Can you work these out from the model? Positions are in its coordinate system, mm. A direction names the side the tool comes from. Coordinates: 2 decimals unless noted, no trailing zeros. Order: outer loops, then holes, each group sorted by start corner. A loop starts at its lowest first (then second) coordinate and runs counter-clockwise, first axis right, second up. Notation, with made-up numbers: (65, 34.25) - (107, 34.25) arc R35 cw to (107, 73.25) - close; hole circle Ø5 at (38.25, 6.25). An arc over 180 degrees is marked (long way). Use a Markdown table: item, result. Add a question column.
(1) We'd pull the mould along X, two halves only. Please class faces 5 (the flat face through (0, -6, 16.51)), 6 (the flat face through (0, 0, 13.97)), 7 (the cylindrical face through (6.49, -10.17, 6.89)), 8 (the cylindrical face through (-1.86, -14.166, 8.139)): pulls with the +X half, pulls with the -X half, needs draft (parallel to the pull), parting line crosses it, or undercut.
(2) I want a section at A-A (x = 0). State how many separate pieces and enclosed holes the cut face has, and give its area (3 significant figures).
(3) If I drill on L1, parallel to Z at x = 0, y = -0.5 (3 decimals); L2, parallel to Y at x = 2, z = 19; L3, parallel to Z at x = -2.75, y = 5.75, over which ranges is the centre line in solid material (lowest first)? Write a range as [from, to].
(4) For pin 1 Ø12 at (x, y) = (4, 2.5) entering from -Z; pin 2 Ø5 at (y, z) = (11, 15.5) entering from -X; pin 3 Ø2 at (x, z) = (-10.5, 6.5) entering from +Y, each with a flat end and sliding along its axis, tell me the tip position at first contact or that it passes through.
(5) I want a section at D-D (y = -11.25). List the corners of the cut face in (x, z) for me.
(6) On a 3-axis mill with a long thin cutter (end or side, diameter ignored), from which of +Z, -Z, +X, -X, +Y, -Y can I reach the whole of each face in a straight line? I mean faces 1 (the cylindrical face through (7.937, 0.072, 24.023)), 2 (the flat face through (-3, -4.762, 22)), 3 (the cylindrical face through (-2.902, 12.563, 12.806)), 4 (the cylindrical face through (-7.937, -0.072, 24.023)). Say none if no direction works.
Autodesk Inventor part; units mm, degrees
ref_plane "Work Plane1" through (0, 14.2875, 0) normal (0, 1, 0) x (-1, 0, 0)
ref_plane "YZ Plane" through (0, 0, 0) normal (1, 0, 0) x (0, 1, 0)
ref_plane "XY Plane" through (0, 0, 0) normal (0, 0, 1) x (1, 0, 0)
sketch "Sketch1" plane through (0, 0, 0) normal (0, 0, 1) x (1, 0, 0)
  circle A0 centre (0, 0) radius 14.2875
  circle A1 centre (0, 0) radius 12.065
  dimension "d0" = 28.575
  dimension "d1" = 24.13
extrude "Extrusion1" add sketch "Sketch1" along normal blind 13.97
sketch "Sketch2" plane through (0, 0, 13.97) normal (0, 0, 1) x (1, 0, 0)
  circle A0 centre (0, 0) radius 14.2875
extrude "Extrusion2" add sketch "Sketch2" along normal blind 2.54
sketch "Sketch3" plane through (0, 0, 16.51) normal (0, 0, 1) x (1, 0, 0)
  circle A0 centre (0, 0) radius 14.2875
  circle A1 centre (0, 0) radius 7.9375
  line L0 (-6.35, -4.7625) -> (6.35, -4.7625)
  line L1 (-6.35, 4.7625) -> (6.35, 4.7625)
  dimension "d6" = 15.875
  dimension "d7" = 9.525
  dimension "d8" = 0
  dimension "d9" = 0
extrude "Extrusion3" add sketch "Sketch3" along normal blind 15.24 contours A1 L0 L1
thread "Thread1"
thread "Thread2"
sketch "Sketch4" plane through (-6.35, 4.7625, 16.51) normal (0, 1, 0) x (1, 0, 0)
  circle A0 centre (6.35, -7.62) radius 3.175
  point P0 (6.35, 16.51)
  dimension "d16" = 6.35
extrude "Extrusion4" cut sketch "Sketch4" against normal blind 15.24
ref_plane "Work Plane1" through (0, 14.2875, 0) normal (0, 1, 0) x (-1, 0, 0)
sketch "Sketch5" plane through (0, 14.2875, 0) normal (0, 1, 0) x (-1, 0, 0)
  line L0 (-14.2875, 16.51) -> (14.2875, 16.51)
  line L1 (-14.2875, 0) -> (14.2875, 0)
  circle A0 centre (0, 8.255) radius 5.3975
  point P0 (0, 0)
  dimension "d20" = 10.795
  dimension "d23" = 8.255
  dimension "d24" = 8.255
extrude "Extrusion5" cut sketch "Sketch5" against normal blind 15.24
properties part number "1in Actuator Bottom Cap 1764"
Answers follow:
| question | item | result |
|---|---|---|
| 1 | face 5 | needs draft |
| 1 | face 6 | undercut |
| 1 | face 7 | undercut |
| 1 | face 8 | parting line crosses it |
| 2 | separate pieces | 3 |
| 2 | enclosed holes | 0 |
| 2 | area | 195 mm² |
| 3 | L1 | z = [13.97, 20.955], [27.305, 31.75] |
| 3 | L2 | y = [-4.76, 4.76] |
| 3 | L3 | z = [13.97, 16.51] |
| 4 | pin 1 | stops at z = 13.97 |
| 4 | pin 2 | stops at x = -11.48 |
| 4 | pin 3 | stops at y = 10.67 |
| 5 | outline | (-8.81, 0) - (-4.36, 0) - (-4.36, 13.97) - (4.36, 13.97) - (4.36, 0) - (8.81, 0) - (8.81, 16.51) - (-8.81, 16.51) - close |
| 6 | face 1 | +Z, +X |
| 6 | face 2 | +Z, +X, -X, -Y |
| 6 | face 3 | +Y |
| 6 | face 4 | +Z, -X |
